from build123d import *

# Parameters (mm, degrees)
F0_W        = 60
F0_H        = 30
F0_R        = 10
F1_DEPTH    = 3
F2_T1_DEPTH = 23
F3_W        = 20
F3_H        = 3
F4_DEPTH    = 25
F5_W        = 20
F5_H        = 3
F6_DEPTH    = 25
F7_R        = 1.75
F8_DEPTH    = 3.0010001


# Not quite as in the source:
# - a fillet or chamfer that OpenCascade refuses, or shapes differently, is made with other operations: its cross-section is extruded or revolved along the edge and cut away or added


with BuildPart() as f1:
    # F0 (on Front) → F1 (new body)
    with BuildSketch(Plane.XZ):
        Rectangle(F0_W, F0_H)
        with Locations((-17.5, 0)):
            Circle(F0_R, mode=Mode.SUBTRACT)
        with BuildLine():
            ThreePointArc((27.5, 0), (17.5, -10), (7.5, 0))
            ThreePointArc((7.5, 0), (17.5, 10), (27.5, 0))
        make_face(mode=Mode.SUBTRACT)
    extrude(amount=F1_DEPTH)

    # F2: fillet of radius 4 on 4 edges, made by hand

    # F2_s2 → F2_t1 (cut)
    with BuildSketch(Plane.XZ.offset(-10)):
        with BuildLine():
            add(Edge.make_bspline(
                [(30, -11), (30, -15), (26, -15)],
                knots=[0, 0, 0, 1, 1, 1], degree=2, weights=[1, 4, 1]))
            Line((26, -15), (30, -15))
            Line((30, -15), (30, -11))
        make_face()
        with BuildLine():
            add(Edge.make_bspline(
                [(-30, -11), (-30, -15), (-26, -15)],
                knots=[0, 0, 0, 1, 1, 1], degree=2, weights=[1, 4, 1]))
            Line((-26, -15), (-30, -15))
            Line((-30, -15), (-30, -11))
        make_face()
        with BuildLine():
            add(Edge.make_bspline(
                [(30, 11), (30, 15), (26, 15)],
                knots=[0, 0, 0, 1, 1, 1], degree=2, weights=[1, 4, 1]))
            Line((26, 15), (30, 15))
            Line((30, 15), (30, 11))
        make_face()
        with BuildLine():
            add(Edge.make_bspline(
                [(-30, 11), (-30, 15), (-26, 15)],
                knots=[0, 0, 0, 1, 1, 1], degree=2, weights=[1, 4, 1]))
            Line((-26, 15), (-30, 15))
            Line((-30, 15), (-30, 11))
        make_face()
    extrude(amount=F2_T1_DEPTH, mode=Mode.SUBTRACT)

    # F3 (on face) → F4 (join)
    with BuildSketch(Plane(origin=(0, 0, -15), x_dir=(1, 0, 0), z_dir=(0, 0, -1))):
        with Locations((0, 1.5)):
            Rectangle(F3_W, F3_H)
    extrude(amount=F4_DEPTH)

    # F5 (on face) → F6 (join)
    with BuildSketch(Plane(origin=(0, 0, 0), x_dir=(-1, 0, 0), z_dir=(0, 1, 0))):
        with Locations((0, -38.5)):
            Rectangle(F5_W, F5_H)
    extrude(amount=F6_DEPTH)

    # F7 (on face) → F8 (cut, through all)
    with BuildSketch(Plane.XY.offset(-37)):
        with Locations((0, 14)):
            Circle(F7_R)
    extrude(amount=-F8_DEPTH, mode=Mode.SUBTRACT)


solid = f1.part
Could you check a few things on this model? Use its own coordinates, in mm. A direction names the side the tool comes from. Coordinates: 2 decimals unless noted, no trailing zeros. Loops run counter-clockwise (first coordinate to the right, second up) from the corner with the lowest first, then second, coordinate; pieces in that order, holes last.
1. Imagine slicing it at C-C (y = 14). Please give me the cut outline in (x, z), and give its area (3 significant figures).
2. Imagine slicing it at B-B (x = 0). Please give me the cut outline in (y, z).
3. Imagine slicing it at A-A (z = 0). Please give me the cut outline in (x, y), and give its area (3 significant figures).
4. For P1, Ø16, axis at x = 3.5, y = 14.5, coming from the +Z side; P2, Ø12, axis at x = -17.5, z = 0, coming from the -Y side; P3, Ø3.5, axis at x = 18.5, y = -1, coming from the -Z side, each with a flat end and sliding along its axis, tell me the tip position at first contact or that it passes through.
5. Imagine slicing it at D-D (z = -8). Please give me the cut outline in (x, y), and give its area (3 significant figures).
6. I need wall thicknesses on L1, parallel to Z at x = -17.5, y = -1.8; L2, parallel to Y at x = 27.5, z = 9; L3, parallel to Y at x = 0, z = -38.1. Which ranges of each line are inside material? Lowest first, please.
7. We'd pull the mould along Z, two halves only. Please class faces 6 (the face through (-2, 12, -37)), 7 (the face through (10, 5, -38)), 8 (the face through (7.96, -1.48, 3)): released by +Z, released by -Z, zero draft, split by the parting line, or undercut.
8. For faces 1 (the face through (0, 0, -5)), 2 (the face through (-18, -1, -15)), 3 (the face through (0, 25, -38)), 4 (the face through (18, -1, -15)), 5 (the face through (-30, -1, 0)), which set-ups out of +Z, -Z, +X, -X, +Y, -Y let a thin tool reach every point of the face, with its end or its side?
Computed values:
1. outline: (-10, -40) - (-1.75, -40) - (-1.75, -37) - (-10, -37) - close; (1.75, -40) - (10, -40) - (10, -37) - (1.75, -37) - close
1. area: 49.5 mm2
2. outline: (-3, -40) - (12.25, -40) - (12.25, -37) - (0, -37) - (0, 15) - (-3, 15) - close; (15.75, -40) - (25, -40) - (25, -37) - (15.75, -37) - close
3. outline: (-30, -3) - (-27.5, -3) - (-27.5, 0) - (-30, 0) - close; (-7.5, -3) - (7.5, -3) - (7.5, 0) - (-7.5, 0) - close; (27.5, -3) - (30, -3) - (30, 0) - (27.5, 0) - close
3. area: 60.0 mm2
4. P1: stops at z = -37
4. P2: passes through
4. P3: stops at z = -15
5. outline: (-30, -3) - (-23.5, -3) - (-23.5, 0) - (-30, 0) - close; (-11.5, -3) - (11.5, -3) - (11.5, 0) - (-11.5, 0) - close; (23.5, -3) - (30, -3) - (30, 0) - (23.5, 0) - close
5. area: 108 mm2
6. L1: z = -15 to -10, 10 to 15
6. L2: y = -3 to 0
6. L3: y = -3 to 12.25, 15.75 to 25
7. face 6: released by +Z
7. face 7: zero draft
7. face 8: undercut
8. face 1: +Z, +X, -X, +Y
8. face 2: -Z, -X, +Y, -Y
8. face 3: +Z, -Z, +X, -X, +Y
8. face 4: -Z, +X, +Y, -Y
8. face 5: +Z, -Z, -X, +Y, -Y
